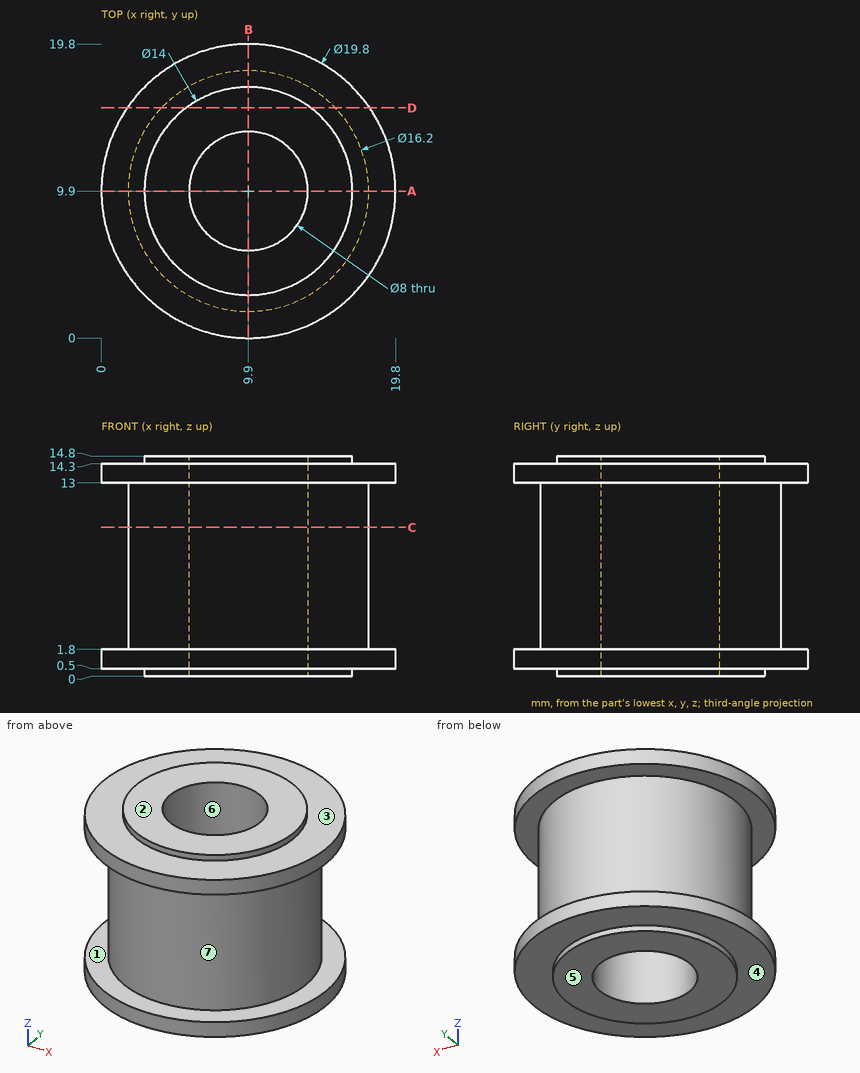
Verification items for this drawing (mm, ordinates from the low corner). A direction names the side the tool comes from. Coordinates: 2 decimals unless noted, no trailing zeros. Loops run counter-clockwise (first coordinate to the right, second up) from the corner with the lowest first, then second, coordinate; pieces in that order, holes last. Notation, with made-up numbers: (-9.75, -19) - (13.25, -19) arc R21 ccw to (13.25, -15) - close; hole circle Ø2 at (15, 7). An arc over 180 degrees is marked (long way). Use one line per item in the form item = value. Start each with the question number.
Item 1: Gauge pin test, flat ends, axial feed: pin 1 (6 mm diameter, centred on y = 14, z = 6, fed in from -X); pin 2 (5 mm diameter, centred on y = 7.5, z = 5, fed in from +X); pin 3 (8 mm diameter, centred on y = 17, z = 2, fed in from -X); pin 4 (5 mm diameter, centred on x = 9.9, y = 9.9, fed in from -Z). Record the tip position at first contact, or that the pin passes through.
Item 2: Section check D-D, the plane y = 15.5. Enter the section's corners in (x, z), and give its area (3 significant figures).
Item 3: Section check A-A, the plane y = 9.9. Enter the section's corners in (x, z).
Item 4: Tool access check on the marked faces 1, 2, 3 and 4. Record the directions out of +Z, -Z, +X, -X, +Y, -Y that give a thin tool (end or side, any length) a straight path to the whole face; none if there is none.
Item 5: Mould release check, pull along X, two halves, no side actions. Record for the marked faces 5, 6 and 7: +X half, -X half, draft (parallel to the pull), parting line (faces both ways), or undercut.
Item 6: Section check C-C, the plane z = 10. Enter the section's corners in (x, y), and give its area (3 significant figures).
Item 7: Thickness scan on probe 1 along Z at (x, y) = (18.5, 11); probe 2 along Y at (x, z) = (9.9, 11.5). Record the ranges inside material, lowest first.
Computed:
q1.pin_1 = 1.88
q1.pin_2 = 18
q1.pin_3 = 0.5
q1.pin_4 = through
q2.outline = (1.74, 0.5) - (5.7, 0.5) - (5.7, 0) - (14.1, 0) - (14.1, 0.5) - (18.06, 0.5) - (18.06, 1.8) - (15.75, 1.8) - (15.75, 13) - (18.06, 13) - (18.06, 14.3) - (14.1, 14.3) - (14.1, 14.8) - (5.7, 14.8) - (5.7, 14.3) - (1.74, 14.3) - (1.74, 13) - (4.05, 13) - (4.05, 1.8) - (1.74, 1.8) - close
q2.area = 182 mm2
q3.outline = (0, 0.5) - (2.9, 0.5) - (2.9, 0) - (5.9, 0) - (5.9, 14.8) - (2.9, 14.8) - (2.9, 14.3) - (0, 14.3) - (0, 13) - (1.8, 13) - (1.8, 1.8) - (0, 1.8) - close; (13.9, 0) - (16.9, 0) - (16.9, 0.5) - (19.8, 0.5) - (19.8, 1.8) - (18, 1.8) - (18, 13) - (19.8, 13) - (19.8, 14.3) - (16.9, 14.3) - (16.9, 14.8) - (13.9, 14.8) - close
q4.face_1 = none
q4.face_2 = +Z, +X, -X, +Y, -Y
q4.face_3 = +Z
q4.face_4 = -Z
q5.face_5 = draft
q5.face_6 = undercut
q5.face_7 = parting line
q6.outline = circle Ø16.2 at (9.9, 9.9); hole circle Ø8 at (9.9, 9.9)
q6.area = 156 mm2
q7.probe_1 = 0.5 to 1.8, 13 to 14.3
q7.probe_2 = 1.8 to 5.9, 13.9 to 18
